Here's the drawing with two shaded views (mm, measured from the low corner). I have some questions. Round coordinates to 2 decimals unless told otherwise and drop trailing zeros. Order: outer loops, then holes, each group sorted by start corner. A loop starts at its lowest first (then second) coordinate and runs counter-clockwise, first axis right, second up.
Q1. If we section it at D-D (z = 24.5): Please give me the cut outline in (x, y), plus the area to 3 significant figures.
Q2. If we section it at A-A (x = 15.5): Please give me the cut outline in (y, z), plus the area to 3 significant figures.
Q3. We'd pull the mould along Z, two halves only. Please class the marked faces 1, 2 and 3: pulls with the +Z half, pulls with the -Z half, needs draft (parallel to the pull), parting line crosses it, or undercut.
Q4. If we section it at B-B (z = 6): Please give me the cut outline in (x, y), plus the area to 3 significant figures.
Q5. If we section it at C-C (y = 14): Please give me the cut outline in (x, z).
Q6. Will this pin go through, and if not, where does the flat tip stop? P1, Ø2, axis at x = 34.5, y = 5, coming from the -Z side.
Q7. If I drill on line 1 (X direction, y = 9, z = 6); line 2 (Z direction, x = 15.5, y = 24.5); line 3 (Z direction, x = 20, y = 13), over which ranges is the centre line in solid material (lowest first)?
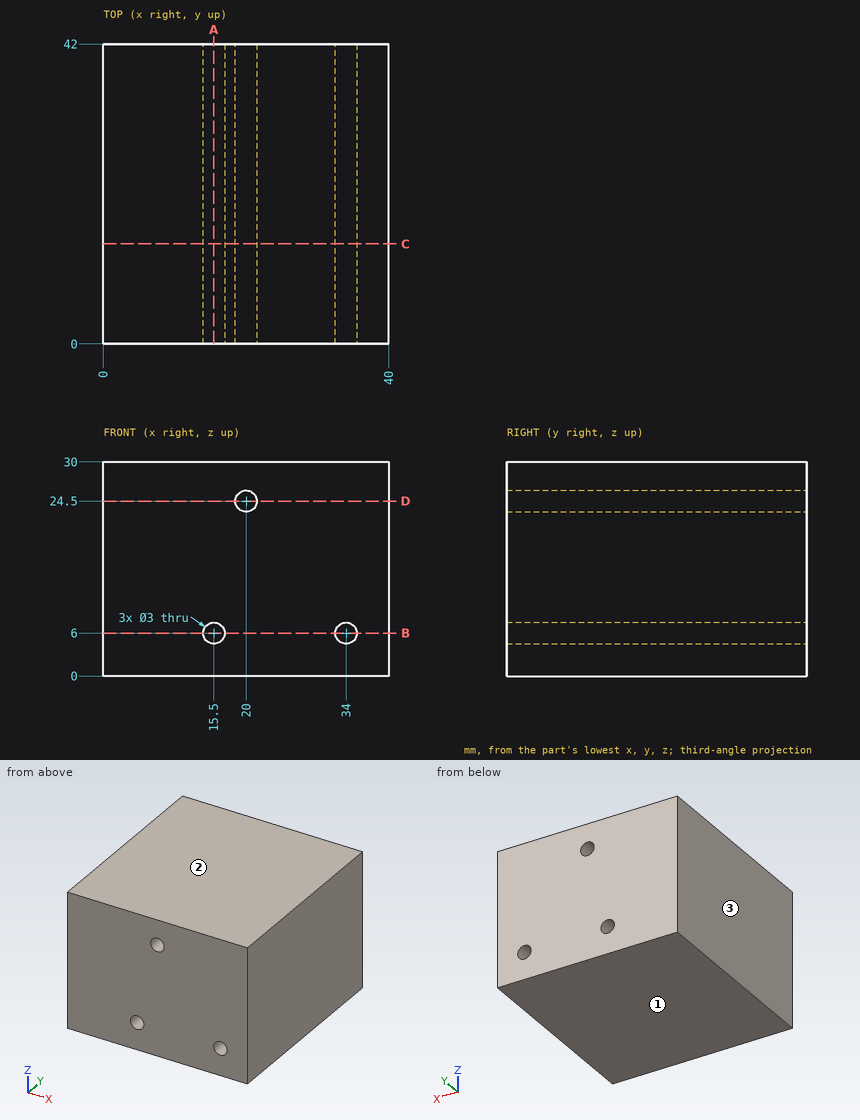
Solution:
1. outline: (0, 0) - (18.5, 0) - (18.5, 42) - (0, 42) - close; (21.5, 0) - (40, 0) - (40, 42) - (21.5, 42) - close
1. area: 1,550 mm2
2. outline: (0, 0) - (42, 0) - (42, 4.5) - (0, 4.5) - close; (0, 7.5) - (42, 7.5) - (42, 30) - (0, 30) - close
2. area: 1,130 mm2
3. face 1: pulls with the -Z half
3. face 2: pulls with the +Z half
3. face 3: needs draft
4. outline: (0, 0) - (14, 0) - (14, 42) - (0, 42) - close; (17, 0) - (32.5, 0) - (32.5, 42) - (17, 42) - close; (35.5, 0) - (40, 0) - (40, 42) - (35.5, 42) - close
4. area: 1,430 mm2
5. outline: (0, 0) - (40, 0) - (40, 30) - (0, 30) - close; hole circle Ø3 at (15.5, 6); hole circle Ø3 at (20, 24.5); hole circle Ø3 at (34, 6)
6. P1: stops at z = 0
7. line 1: x = 0 to 14, 17 to 32.5, 35.5 to 40
7. line 2: z = 0 to 4.5, 7.5 to 30
7. line 3: z = 0 to 23, 26 to 30
